Verification items for this drawing (mm, ordinates from the low corner). Give positions to 0.01 mm unless a question says otherwise; leave off trailing zeros. Write each loop counter-clockwise with the first axis right and the second up, starting at its lowest first coordinate (ties: lowest second). Pieces come first, ordered by that corner, then holes. Notation, with made-up numbers: (66, 7.5) -> (118, 7.5) arc R32 ccw to (118, 41.5) -> close; hole circle Ø6 at (47.25, -38). An arc over 180 degrees is marked (long way). Write item = value, one per line.
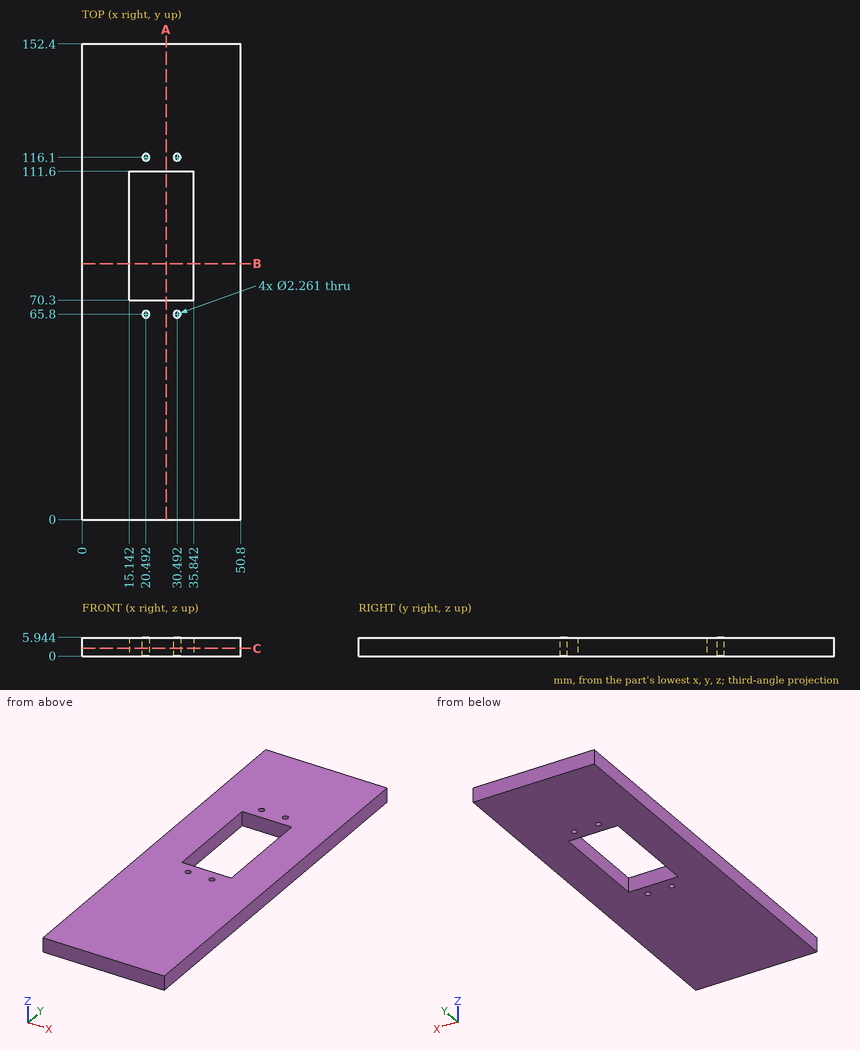
Item 1: Go/stop test with a flat-tipped pin: P1, Ø2, axis at x = 20.49, y = 65.8, coming from the -Z side. Record where the tip stops, or that it passes through.
Response values:
P1 = through
Item 2: Material ranges on line 1 (X direction, y = 66, z = 5.5) (1 decimal); line 2 (Y direction, x = 24, z = 2.4); line 3 (Y direction, x = 30, z = 1.25), recorded low to high.
Response values:
line_1 = 0 to 19.4, 21.6 to 29.4, 31.6 to 50.8
line_2 = 0 to 70.3, 111.6 to 152.4
line_3 = 0 to 64.78, 66.82 to 70.3, 111.6 to 115.08, 117.12 to 152.4
Item 3: Sectioned sample at C-C on z = 2.45. Record the cut outline in (x, y), then the cut area to 3 significant figures.
Response values:
outline = (0, 0) -> (50.8, 0) -> (50.8, 152.4) -> (0, 152.4) -> close; hole (15.14, 70.3) -> (35.84, 70.3) -> (35.84, 111.6) -> (15.14, 111.6) -> close; hole circle Ø2.26 at (20.49, 65.8); hole circle Ø2.26 at (20.49, 116.1); hole circle Ø2.26 at (30.49, 65.8); hole circle Ø2.26 at (30.49, 116.1)
area = 6,870 mm^2
Item 4: Sectioned sample at A-A on x = 27. Record the cut outline in (y, z).
Response values:
outline = (0, 0) -> (70.3, 0) -> (70.3, 5.94) -> (0, 5.94) -> close; (111.6, 0) -> (152.4, 0) -> (152.4, 5.94) -> (111.6, 5.94) -> close
Item 5: Sectioned sample at B-B on y = 82. Record the cut outline in (x, z), then the cut area to 3 significant figures.
Response values:
outline = (0, 0) -> (15.14, 0) -> (15.14, 5.94) -> (0, 5.94) -> close; (35.84, 0) -> (50.8, 0) -> (50.8, 5.94) -> (35.84, 5.94) -> close
area = 179 mm^2
